Part model, mm, in its own coordinate system. A direction names the side the tool comes from. Give positions to 0.01 mm unless a question says otherwise; leave off trailing zeros. Write each loop counter-clockwise with the first axis right and the second up, starting at its lowest first coordinate (ties: lowest second). Pieces come first, ordered by that corner, then holes.
```python
from build123d import *

# Parameters (mm, degrees)
F0_R     = 38.1
F1_DEPTH = 7.62
F2_R     = 11.8491
F3_DEPTH = 7.621
F4_SIZE  = 0.889
F5_R     = 2.286
F6_DEPTH = 5.08
F7_SIZE  = 0.508
F8_R     = 18.1991
F8_R_2   = 11.8491
F9_DEPTH = 12.7
F10_R    = 2.032
F11_SIZE = 2.54


with BuildPart() as f1:
    # F0 (on Top) → F1 (new body)
    with BuildSketch(Plane.XY):
        Circle(F0_R)
    extrude(amount=F1_DEPTH)

    # F2 (on face) → F3 (cut, through all)
    with BuildSketch(Plane.XY.offset(7.62)):
        Circle(F2_R)
    extrude(amount=-F3_DEPTH, mode=Mode.SUBTRACT)

    # F4
    f4_edges = [f1.edges().sort_by_distance(p)[0] for p in [
        (-38.1, 0, 7.62),
        (-11.8491, 0, 0),
    ]]
    chamfer(f4_edges, length=F4_SIZE)

    # F5 (on face) → F6 (join)
    with BuildSketch(Plane(origin=(0, 0, 0), x_dir=(1, 0, 0), z_dir=(0, 0, -1))):
        with Locations((-33.4009492, 0)):
            Circle(F5_R)
        with Locations((33.4009492, 0)):
            Circle(F5_R)
    extrude(amount=F6_DEPTH)

    # F7
    f7_edges = [f1.edges().sort_by_distance(p)[0] for p in [
        (31.114949, 0, -5.08),
        (-35.686949, 0, -5.08),
    ]]
    chamfer(f7_edges, length=F7_SIZE)

    # F8 (on face) → F9 (join)
    with BuildSketch(Plane.XY.offset(7.62)):
        Circle(F8_R)
        Circle(F8_R_2, mode=Mode.SUBTRACT)
    extrude(amount=F9_DEPTH)

    # F10
    f10_edges = [f1.edges().sort_by_distance(p)[0] for p in [
        (-11.8491, 0, 7.62),
        (11.8491, 0, 4.2545),
        (-11.8491, 0, 0.889),
        (11.8491, 0, 13.97),
        (-11.8491, 0, 20.32),
    ]]
    fillet(f10_edges, radius=F10_R)

    # F11
    f11_edges = [f1.edges().sort_by_distance(p)[0] for p in [
        (-18.1991, 0, 20.32),
    ]]
    chamfer(f11_edges, length=F11_SIZE)


solid = f1.part
```
1) Pin check, flat tips, straight feed: pin 1 Ø12 at (x, y) = (-22.5, 15.5) entering from -Z; pin 2 Ø2 at (x, z) = (-18.5, 6.5) entering from -Y; pin 3 Ø1.5 at (x, z) = (11.5, 17.5) entering from +Y. Stop position of each tip, or through.
Answers follow:
pin 1: stops at z = 0
pin 2: stops at y = -33.84
pin 3: stops at y = 14.68
2) Wall check: L1, parallel to Y at x = 0, z = 15.25; L2, parallel to X at y = 0.5, z = 2.25; L3, parallel to Z at x = -8, y = 11.5. Give the ranges that are in metal, low to high.
Answers follow:
L1: y = -18.2 to -11.85, 11.85 to 18.2
L2: x = -38.1 to -11.84, 11.84 to 38.1
L3: z = 0 to 20.32
3) 3-axis set-ups, long thin cutter, end or side, ignore diameter. For faces 4 (the face through (-31.3, 0.9, -2.3)), 5 (the face through (16, 9, 7.62)), 6 (the face through (33, 0, -5.08)): which of +Z, -Z, +X, -X, +Y, -Y reach the whole face in a straight line?
Answers follow:
face 4: -Z
face 5: +Z
face 6: -Z, +X, -X, +Y, -Y
4) Saw through at B-B, the plane z = -2.75. Write the cut outline in (x, y).
Answers follow:
outline: circle Ø4.57 at (-33.4, 0); circle Ø4.57 at (33.4, 0)
5) Two-plate mould, pull along X, no slides. Class faces 1 (the face through (-1, -14, 20.32)), 2 (the face through (35.58, -0.69, -2.25)), 3 (the face through (17.359, 5.467, 12.629)): +X half, -X half, draft (parallel to the pull), parting line (faces both ways), or undercut.
Answers follow:
face 1: draft
face 2: undercut
face 3: parting line
6) Saw through at A-A, the plane z = 5.75. Write the cut outline in (x, y).
Answers follow:
outline: circle Ø76.2 at (0, 0); hole circle Ø23.7 at (0, 0)
